```python
from build123d import *

# Parameters (mm, degrees)
SKETCH1_R               = 1.5
BOSS_EXTRUDE1_DEPTH     = 3
SKETCH3_W               = 4.615398666
SKETCH3_H               = 10
BOSS_EXTRUDE2_DEPTH     = 12.9997796
FILLET7_R               = 1
CUT_EXTRUDE4_DEPTH      = 10
SKETCH9_W               = 13.564457496
SKETCH9_H               = 20
SKETCH9_R               = 1.5
BOSS_EXTRUDE3_DEPTH     = 3
CHAMFER1_SIZE           = 10
CHAMFER2_SIZE           = 10
FILLET8_R               = 4
CUT_EXTRUDE5_DEPTH      = 27.355587635
CUT_EXTRUDE5_DEPTH_BACK = 27.355587635
SKETCH10_W              = 8.131195533
SKETCH10_H              = 6.749631571
SKETCH10_H_2            = 7.013496214


with BuildPart() as part:
    # Sketch1 → Boss-Extrude1 (new body)
    with BuildSketch(Plane(origin=(0, 0, 0), x_dir=(1, 0, 0), z_dir=(0, 1, 0))):
        Polygon((-3, -11.32792047), (3, -11.32792047), (3, -5), (7.615398666, -5), (7.615398666, 5), (3, 5), (3, 11.32792047), (-3, 11.32792047), align=None)
        with Locations(Location((0, 8.5, 0), (0, 0, 270))):
            Circle(SKETCH1_R, mode=Mode.SUBTRACT)
        with Locations(Location((0, -8.5, 0), (0, 0, 270))):
            Circle(SKETCH1_R, mode=Mode.SUBTRACT)
    extrude(amount=BOSS_EXTRUDE1_DEPTH)

    # Sketch3 → Boss-Extrude2 (add)
    with BuildSketch(Plane(origin=(0, 3, 0), x_dir=(1, 0, 0), z_dir=(0, 1, 0))):
        with Locations((5.307699333, 0)):
            Rectangle(SKETCH3_W, SKETCH3_H)
    extrude(amount=BOSS_EXTRUDE2_DEPTH)

    # Fillet7
    fillet7_edges = [part.edges().sort_by_distance(p)[0] for p in [
        (3, 1.5, 11.32792047),
        (3, 1.5, -11.32792047),
    ]]
    fillet(fillet7_edges, radius=FILLET7_R)

    # Sketch7 → Cut-Extrude4 (cut)
    with BuildSketch(Plane.XZ):
        with BuildLine():
            Line((-3.65526474, -6.392053518), (-3.78188192, 6.478485425))
            ThreePointArc((-3.78188192, 6.478485425), (-0.319780446, 0.076652438), (-3.65526474, -6.392053518))
        make_face()
    extrude(amount=-CUT_EXTRUDE4_DEPTH, mode=Mode.SUBTRACT)

    # Sketch9 → Boss-Extrude3 (add)
    with BuildSketch(Plane(origin=(0, 15.9997796, 0), x_dir=(1, 0, 0), z_dir=(0, 1, 0))):
        with Locations((10.833169918, 0)):
            Rectangle(SKETCH9_W, SKETCH9_H)
        with Locations(Location((12.615398666, 6, 0), (0, 0, 270))):
            Circle(SKETCH9_R, mode=Mode.SUBTRACT)
        with Locations(Location((12.615398666, -6, 0), (0, 0, 270))):
            Circle(SKETCH9_R, mode=Mode.SUBTRACT)
    extrude(amount=BOSS_EXTRUDE3_DEPTH)

    # Chamfer1
    # the kernel refuses this chamfer: 10 mm, written as the material it adds along each edge
    with BuildSketch(Plane(origin=(4.05094117, 15.9997796, 5), x_dir=(0, -0.9996219169112968, -0.027495876610586403), z_dir=(1, 0, 0))) as chamfer1_piece_1_section:
        Polygon((CHAMFER1_SIZE * 0.999621916911, -CHAMFER1_SIZE * 0.0274958766106), (-CHAMFER1_SIZE * 0.0274958766106, -CHAMFER1_SIZE * 0.999621916911), (0, 0), align=None)
    chamfer1_piece_1 = extrude(amount=3.564457497, mode=Mode.PRIVATE)
    chamfer1_piece_1 = split(chamfer1_piece_1, bisect_by=Plane(origin=(5.833169918, 12.110890711, 10), z_dir=(0, 0, -1)), keep=Keep.TOP, mode=Mode.PRIVATE)
    add(chamfer1_piece_1)

    # Chamfer2
    # the kernel refuses this chamfer: 10 mm, written as the material it adds along each edge
    with BuildSketch(Plane(origin=(7.615398666, 15.9997796, -5), x_dir=(0, -0.9996219169112968, 0.027495876610586403), z_dir=(-1, 0, 0))) as chamfer2_piece_1_section:
        Polygon((CHAMFER2_SIZE * 0.999621916911, -CHAMFER2_SIZE * 0.0274958766106), (-CHAMFER2_SIZE * 0.0274958766106, -CHAMFER2_SIZE * 0.999621916911), (0, 0), align=None)
    chamfer2_piece_1 = extrude(amount=3.564457497, mode=Mode.PRIVATE)
    chamfer2_piece_1 = split(chamfer2_piece_1, bisect_by=Plane(origin=(5.833169918, 12.110890711, -10), z_dir=(0, 0, 1)), keep=Keep.TOP, mode=Mode.PRIVATE)
    add(chamfer2_piece_1)

    # Fillet8
    fillet8_edges = [part.edges().sort_by_distance(p)[0] for p in [
        (3, 3, 0),
    ]]
    fillet(fillet8_edges, radius=FILLET8_R)

    # Sketch10 → Cut-Extrude5 (cut, two sides: drawn at the far end of the back side and taken through both)
    with BuildSketch(Plane(origin=(0, 3, 0), x_dir=(1, 0, 0), z_dir=(0, 1, 0)).offset(-CUT_EXTRUDE5_DEPTH_BACK)):
        with Locations((1.065597767, 9.256059268)):
            Rectangle(SKETCH10_W, SKETCH10_H)
        with Locations((1.065597767, -9.38799159)):
            Rectangle(SKETCH10_W, SKETCH10_H_2)
    extrude(amount=CUT_EXTRUDE5_DEPTH + CUT_EXTRUDE5_DEPTH_BACK, mode=Mode.SUBTRACT)


solid = part.part
```
Here's how the part is built. I have some questions about the finished solid (model axes, mm). A direction names the side the tool comes from. Give positions to 0.01 mm unless a question says otherwise; leave off trailing zeros. Order: outer loops, then holes, each group sorted by start corner. A loop starts at its lowest first (then second) coordinate and runs counter-clockwise, first axis right, second up. Notation, with made-up numbers: (43.25, 89.5) - (57.25, 89.5) arc R21 ccw to (57.25, 102.5) - close; hole circle Ø5 at (2.25, 18). An arc over 180 degrees is marked (long way). Answer as a JSON object with one key per item and string values. Group by question number.
Item 1: If we section it at A-A on z = 7: Please give me the cut outline in (x, y), and give its area (3 significant figures).
Item 2: If we mould it in two halves opening along Z, with no side actions, what happens to faces 5 (the flat face through (0, 3, 5.4)), 6 (the cylindrical face through (12.68, 17.48, -7.5)), 7 (the flat face through (0, 1, 5.881))? For each: pulls with the +Z half, pulls with the -Z half, needs draft (parallel to the pull), parting line crosses it, or undercut.
Item 3: Please list where these lines run through material, in increasing order: probe 1 along X at (y, z) = (17.9, -6); probe 2 along X at (y, z) = (17.75, 8); probe 3 along Y at (x, z) = (13.75, 3).
Item 4: Which directions (+Z, -Z, +X, -X, +Y, -Y) give clear straight access to the entire face, cutting with the end or side of a thin tool? Please do faces 1 (the flat face through (5.131, 14, 8)), 2 (the flat face through (13, 16, 0)), 3 (the flat face through (5.131, 14, -8)), 4 (the flat face through (3, 11, 0)).
Item 5: If we section it at B-B on y = 1.75: Please give me the cut outline in (x, z), and give its area (3 significant figures).
Item 6: For P1, Ø2.5, axis at x = 0, y = 1.5, coming from the +Z side; P2, Ø0.5, axis at x = 4.5, y = 11.5, coming from the -Z side; P3, Ø2.5, axis at y = 11, z = -1.5, coming from the -X side, each with a flat end and sliding along its axis, tell me the tip position at first contact or that it passes through.
Item 7: If we section it at D-D on y = 15.5: Please give me the cut outline in (x, z).
Item 8: If we section it at C-C on x = 15.75: Please give me the cut outline in (y, z).
Result set:
{
 "1": {"outline": "(5.13, 8) - (7.62, 8) - (7.62, 16) - (11.5, 16) - (11.5, 19) - (5.13, 19) - close; (13.73, 16) - (17.62, 16) - (17.62, 19) - (13.73, 19) - close", "area": "50.6 mm²"},
 "2": {"face 5": "needs draft", "face 6": "undercut", "face 7": "pulls with the +Z half"},
 "3": {"probe 1": "5.13 to 11.12, 14.12 to 17.62", "probe 2": "5.13 to 17.62", "probe 3": "16 to 19"},
 "4": {"face 1": "+Z, -X, +Y, -Y", "face 2": "+Z, -Z, +X, -Y", "face 3": "-Z, -X, +Y, -Y", "face 4": "+Z, -Z, -X, +Y"},
 "5": {"outline": "(-3, -5.88) - (3, -5.88) - (3, -5) - (7.62, -5) - (7.62, 5) - (3, 5) - (3, 5.88) - (-3, 5.88) arc R7.79 cw to start", "area": "94.9 mm²"},
 "6": {"P1": "z = 5.88", "P2": "z = -5.88", "P3": "x = 3"},
 "7": {"outline": "(3, -5) - (4.05, -5) - (4.05, -5.88) - (5.13, -5.88) - (5.13, -10) - (7.62, -10) - (7.62, 10) - (5.13, 10) - (5.13, 5.88) - (4.05, 5.88) - (4.05, 5) - (3, 5) - close"},
 "8": {"outline": "(16, -10) - (19, -10) - (19, 10) - (16, 10) - close"}
}
